```python
from build123d import *

# Parameters (mm, degrees)
SKETCH1_W           = 69.85
SKETCH1_H           = 44.45
SKETCH1_R           = 1.25
SKETCH1_R_2         = 3.2639
BOSS_EXTRUDE1_DEPTH = 1
SKETCH2_R           = 4
SKETCH2_R_2         = 1.51
BOSS_EXTRUDE2_DEPTH = 8.525


with BuildPart() as part:
    # Sketch1 → Boss-Extrude1 (new body)
    with BuildSketch(Plane(origin=(0, 0, 0), x_dir=(1, 0, 0), z_dir=(0, 1, 0))):
        with Locations((34.925, 22.225)):
            Rectangle(SKETCH1_W, SKETCH1_H)
        with Locations((24.925, 12.225)):
            Circle(SKETCH1_R, mode=Mode.SUBTRACT)
        with Locations((34.925, 12.225)):
            Circle(SKETCH1_R, mode=Mode.SUBTRACT)
        with Locations((44.925, 12.225)):
            Circle(SKETCH1_R, mode=Mode.SUBTRACT)
        with Locations((24.925, 32.225)):
            Circle(SKETCH1_R, mode=Mode.SUBTRACT)
        with Locations((24.925, 22.225)):
            Circle(SKETCH1_R, mode=Mode.SUBTRACT)
        with Locations((34.925, 32.225)):
            Circle(SKETCH1_R, mode=Mode.SUBTRACT)
        with Locations((44.925, 32.225)):
            Circle(SKETCH1_R, mode=Mode.SUBTRACT)
        with Locations((44.925, 22.225)):
            Circle(SKETCH1_R, mode=Mode.SUBTRACT)
        with Locations((34.925, 22.225)):
            Circle(SKETCH1_R, mode=Mode.SUBTRACT)
        with Locations((60.325, 9.525)):
            Circle(SKETCH1_R_2, mode=Mode.SUBTRACT)
        with Locations((9.525, 9.525)):
            Circle(SKETCH1_R_2, mode=Mode.SUBTRACT)
        with Locations((60.325, 34.925)):
            Circle(SKETCH1_R_2, mode=Mode.SUBTRACT)
        with Locations((9.525, 34.925)):
            Circle(SKETCH1_R_2, mode=Mode.SUBTRACT)
    extrude(amount=BOSS_EXTRUDE1_DEPTH)

    # Sketch2 → Boss-Extrude2 (add)
    with BuildSketch(Plane(origin=(0, 1, 0), x_dir=(1, 0, 0), z_dir=(0, 1, 0))):
        with Locations((34.925, 22.225)):
            Circle(SKETCH2_R)
        with Locations((34.925, 22.225)):
            Circle(SKETCH2_R_2, mode=Mode.SUBTRACT)
        with Locations((44.925, 22.225)):
            Circle(SKETCH2_R)
        with Locations((44.925, 22.225)):
            Circle(SKETCH2_R_2, mode=Mode.SUBTRACT)
        with Locations((44.925, 32.225)):
            Circle(SKETCH2_R)
        with Locations((44.925, 32.225)):
            Circle(SKETCH2_R_2, mode=Mode.SUBTRACT)
        with Locations((34.925, 32.225)):
            Circle(SKETCH2_R)
        with Locations((34.925, 32.225)):
            Circle(SKETCH2_R_2, mode=Mode.SUBTRACT)
        with Locations((44.925, 12.225)):
            Circle(SKETCH2_R)
        with Locations((44.925, 12.225)):
            Circle(SKETCH2_R_2, mode=Mode.SUBTRACT)
        with Locations((34.925, 12.225)):
            Circle(SKETCH2_R)
        with Locations((34.925, 12.225)):
            Circle(SKETCH2_R_2, mode=Mode.SUBTRACT)
        with Locations((24.925, 22.225)):
            Circle(SKETCH2_R)
        with Locations((24.925, 22.225)):
            Circle(SKETCH2_R_2, mode=Mode.SUBTRACT)
        with Locations((24.925, 32.225)):
            Circle(SKETCH2_R)
        with Locations((24.925, 32.225)):
            Circle(SKETCH2_R_2, mode=Mode.SUBTRACT)
        with Locations((24.925, 12.225)):
            Circle(SKETCH2_R)
        with Locations((24.925, 12.225)):
            Circle(SKETCH2_R_2, mode=Mode.SUBTRACT)
    extrude(amount=BOSS_EXTRUDE2_DEPTH)


solid = part.part
```
For this review, take the finished solid that the model builds, in its own axes (mm). A direction names the side the tool comes from. Round coordinates to 2 decimals unless told otherwise and drop trailing zeros. Order: outer loops, then holes, each group sorted by start corner. A loop starts at its lowest first (then second) coordinate and runs counter-clockwise, first axis right, second up.
Q1. We need section B-B, the plane z = -17. Give the boundary of the cut face in (x, y).
Findings below:
outline: (0, 0) - (69.85, 0) - (69.85, 1) - (0, 1) - close
Q2. Insertion check: P1, Ø3.5, axis at x = 35, z = -22, coming from the +Y side (3 decimals); P2, Ø2, axis at x = 24.925, z = -12.225, coming from the +Y side; P3, Ø1.5, axis at x = 34.5, y = 7, coming from the -Z side (3 decimals); P4, Ø1.5, axis at x = 25.5, z = -22.5, coming from the +Y side. Each pin has a flat end and moves straight along its axis. Give the tip position at first contact, or say it passes through.
Findings below:
P1: stops at y = 9.525
P2: passes through
P3: stops at z = -36.225
P4: stops at y = 1
Q3. Machinability: for faces 1 (the cylindrical face through (33.812, 5.203, -23.246)), 2 (the flat face through (34.9, 9.525, -10.5)), which of the approach directions +Z, -Z, +X, -X, +Y, -Y give a long, thin tool a straight path to every point of the face, cutting with its end or side? Answer none if there is none.
Findings below:
face 1: +Y
face 2: +Z, -Z, +X, -X, +Y
Q4. We need section D-D, the plane x = 54. Give the boundary of the cut face in (y, z).
Findings below:
outline: (0, -44.45) - (1, -44.45) - (1, 0) - (0, 0) - close
Q5. We need section A-A, the plane y = 5.75. State how many separate pieces and enclosed holes the cut face has, plus the area to 3 significant figures.
Findings below:
separate pieces: 9
enclosed holes: 9
area: 388 mm2
Q6. Mouldability with a two-part tool opening along Z and no side actions: class faces 3 (the flat face through (34, 0, -27)), 4 (the cylindrical face through (46.771, 5.203, -18.676)) as pulls with the +Z half, pulls with the -Z half, needs draft (parallel to the pull), parting line crosses it, or undercut.
Findings below:
face 3: needs draft
face 4: undercut
Q7. We need section C-C, the plane x = 37.5. Give the boundary of the cut face in (y, z) (3 decimals).
Findings below:
outline: (0, -44.45) - (1, -44.45) - (1, -35.286) - (9.525, -35.286) - (9.525, -29.164) - (1, -29.164) - (1, -25.286) - (9.525, -25.286) - (9.525, -19.164) - (1, -19.164) - (1, -15.286) - (9.525, -15.286) - (9.525, -9.164) - (1, -9.164) - (1, 0) - (0, 0) - close
Q8. Wall thickness on line 1 (Z direction, x = 24, y = 6.75); line 2 (X direction, y = 7, z = -23.5); line 3 (Z direction, x = 43, y = 3): over which ranges is each line inside the solid? List them lowest first.
Findings below:
line 1: z = -36.12 to -33.42, -31.03 to -28.33, -26.12 to -23.42, -21.03 to -18.33, -16.12 to -13.42, -11.03 to -8.33
line 2: x = 21.13 to 24.12, 25.73 to 28.72, 31.13 to 34.12, 35.73 to 38.72, 41.13 to 44.12, 45.73 to 48.72
line 3: z = -35.73 to -28.72, -25.73 to -18.72, -15.73 to -8.72
